Check sheet for the modelled part. Datum: model origin and axes. Units: mm. Give positions to 0.01 mm unless a question says otherwise; leave off trailing zeros. Write each loop counter-clockwise with the first axis right and the second up, starting at its lowest first coordinate (ties: lowest second). Pieces come first, ordered by that corner, then holes. Notation, with made-up numbers: (49.25, -4) -> (99.25, -4) arc R9 cw to (99.25, 8) -> close; hole circle Ø6 at (64.5, -15). An arc over 180 degrees is marked (long way). Answer as a JSON object with one key per item and string values.
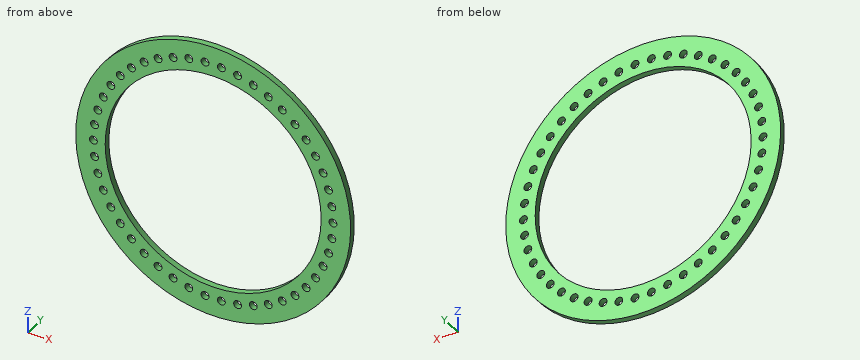
from build123d import *

# Parameters (mm, degrees)
SKETCH1_R           = 35
SKETCH1_R_2         = 27.5
BOSS_EXTRUDE1_DEPTH = 1.5
SKETCH2_R           = 1
CUT_EXTRUDE1_DEPTH  = 1.5
CIRPATTERN1_COUNT   = 46


with BuildPart() as part:
    # Sketch1 → Boss-Extrude1 (new body)
    with BuildSketch(Plane(origin=(0, 0, 0), x_dir=(1, 0, 0), z_dir=(0, 1, 0))):
        with Locations(Location((0, 0, 0), (0, 0, 270))):
            Circle(SKETCH1_R)
        with Locations(Location((0, 0, 0), (0, 0, 270))):
            Circle(SKETCH1_R_2, mode=Mode.SUBTRACT)
    extrude(amount=BOSS_EXTRUDE1_DEPTH)

    # Sketch2 → Cut-Extrude1 (cut)
    with BuildSketch(Plane(origin=(0, 1.5, 0), x_dir=(1, 0, 0), z_dir=(0, 1, 0))):
        with Locations(Location((30.5, 0, 0), (0, 0, 270))):
            Circle(SKETCH2_R)
    cut_extrude1 = extrude(amount=-CUT_EXTRUDE1_DEPTH, mode=Mode.SUBTRACT)

    # CirPattern1: Cut-Extrude1 ×46 about axis
    cirpattern1_axis = Axis((0, 0, 0), (0, 1, 0))
    for i in range(1, CIRPATTERN1_COUNT):
        add(cut_extrude1.rotate(cirpattern1_axis, i * 360 / CIRPATTERN1_COUNT), mode=Mode.SUBTRACT)


solid = part.part
1. Sectioned sample at B-B, the plane z = 0. Enter the section's corners in (x, y).
Determined:
{"outline": "(-35, 0) -> (-31.5, 0) -> (-31.5, 1.5) -> (-35, 1.5) -> close; (-29.5, 0) -> (-27.5, 0) -> (-27.5, 1.5) -> (-29.5, 1.5) -> close; (27.5, 0) -> (29.5, 0) -> (29.5, 1.5) -> (27.5, 1.5) -> close; (31.5, 0) -> (35, 0) -> (35, 1.5) -> (31.5, 1.5) -> close"}
2. Sectioned sample at A-A, the plane x = 0. Enter the section's corners in (y, z), plus the area to 3 significant figures.
Determined:
{"outline": "(0, -35) -> (1.5, -35) -> (1.5, -27.5) -> (0, -27.5) -> close; (0, 27.5) -> (1.5, 27.5) -> (1.5, 35) -> (0, 35) -> close", "area": "22.5 mm^2"}
3. Scan lines: L1, parallel to X at y = 1.1, z = -19.5; L2, parallel to Z at x = 1, y = 0.5; L3, parallel to X at y = 0.5, z = -19. Record each from-to range of solid material in increasing order. Write a range as [from, to].
Determined:
{"L1": "[-29.06, -24.63], [-22.69, -19.39], [19.39, 22.69], [24.63, 29.06]", "L2": "[-34.99, -27.48], [27.48, 34.99]", "L3": "[-29.39, -24.63], [-22.69, -19.88], [19.88, 22.69], [24.63, 29.39]"}
4. Go/stop test with a flat-tipped pin: P1, Ø1.8, axis at x = -26.06, z = -15.85, coming from the -Y side. Record where the tip stops, or that it passes through.
Determined:
{"P1": "through"}
5. Sectioned sample at C-C, the plane y = 1.1. State how many separate pieces and enclosed holes the cut face has, plus the area to 3 significant figures.
Determined:
{"separate pieces": "1", "enclosed holes": "47", "area": "1,330 mm^2"}
